```python
from build123d import *

# Parameters (mm, degrees)
EXTRUDE_1_DEPTH              = 88
HOLE_WIZARD_M4_1_D           = 4.5
HOLE_WIZARD_M4_1_CBORE_D     = 8
HOLE_WIZARD_M4_1_CBORE_DEPTH = 4.4
HOLE_WIZARD_M4_1_2_D         = 3.3
HOLE_WIZARD_M3_1_D           = 2.5
HOLE_WIZARD_M3_1_DEPTH       = 9.5
HOLE_WIZARD_M3_1_TIP         = 0.751075774
SKETCH_8_R                   = 1.75
CUT_EXTRUDE_1_DEPTH          = 5


with BuildPart() as part:
    # 草图1 → 凸台-拉伸1 (new body)
    with BuildSketch(Plane.XY):
        Polygon((-9, 10), (-9, 5), (-74, 5), (-74, 12), (-79, 12), (-79, 5.9), (-79.6, 5.9), (-79.6, 0), (0, 0), (0, 10), (-2, 10), (-2, 8), (-7, 8), (-7, 10), align=None)
    extrude(amount=EXTRUDE_1_DEPTH)

    # Hole Wizard M4 _1 (through all)
    with Locations(Plane(origin=(0, 0, 0), x_dir=(-1, 0, 0), z_dir=(0, -1, 0))):
        with Locations((4.5, -11.5), (4.5, -44), (4.5, -76.5)):
            CounterBoreHole(HOLE_WIZARD_M4_1_D / 2, HOLE_WIZARD_M4_1_CBORE_D / 2, HOLE_WIZARD_M4_1_CBORE_DEPTH)

    # Hole Wizard M4 _1 2 (through all)
    with Locations(Plane(origin=(0, 0, 0), x_dir=(-1, 0, 0), z_dir=(0, -1, 0))):
        with Locations((68.8, -14), (68.8, -22)):
            Hole(HOLE_WIZARD_M4_1_2_D / 2)

    # M3 螺纹孔1
    with Locations(Plane.ZY.offset(79.6)):
        with Locations((11.5, 3), (44, 3), (76.5, 3)):
            Hole(HOLE_WIZARD_M3_1_D / 2, depth=HOLE_WIZARD_M3_1_DEPTH)
            with Locations((0, 0, -(HOLE_WIZARD_M3_1_DEPTH + HOLE_WIZARD_M3_1_TIP / 2))):  # 118° drill point
                Cone(0, HOLE_WIZARD_M3_1_D / 2, HOLE_WIZARD_M3_1_TIP, mode=Mode.SUBTRACT)

    # 草图8 → 切除-拉伸1 (cut)
    with BuildSketch(Plane.ZY.offset(79)):
        with Locations((63, 9.5)):
            Circle(SKETCH_8_R)
    extrude(amount=-CUT_EXTRUDE_1_DEPTH, mode=Mode.SUBTRACT)


solid = part.part
```
Work out the finished part from the listing and answer in its coordinate system (mm). A direction names the side the tool comes from. Coordinates: 2 decimals unless noted, no trailing zeros. Write each loop counter-clockwise with the first axis right and the second up, starting at its lowest first coordinate (ties: lowest second). Pieces come first, ordered by that corner, then holes. Notation, with made-up numbers: (42.25, -38) - (70.25, -38) arc R14 cw to (70.25, -28) - close; hole circle Ø2 at (9, -13.5). An arc over 180 degrees is marked (long way). Answer as a JSON object with one key per item and string values.
Q1. Find section B-B (z = 34). Write down the section's boundary in (x, y), plus the area to 3 significant figures.
Results list:
{"outline": "(-79.6, 0) - (0, 0) - (0, 10) - (-2, 10) - (-2, 8) - (-7, 8) - (-7, 10) - (-9, 10) - (-9, 5) - (-74, 5) - (-74, 12) - (-79, 12) - (-79, 5.9) - (-79.6, 5.9) - close", "area": "469 mm^2"}
Q2. Consider L1, parallel to Z at x = -4.5, y = 6.2; L2, parallel to Z at x = -68.8, y = 2.05; L3, parallel to X at y = 8.25, z = 74. Determine where each line is inside the solid, lowest interval first. Write a range as from..to.
Results list:
{"L1": "z = 0..9.25, 13.75..41.75, 46.25..74.25, 78.75..88", "L2": "z = 0..12.35, 15.65..20.35, 23.65..88", "L3": "x = -79..-74, -9..-7, -2..0"}
Q3. For a pull along Z with two mould halves and no side action, classify faces 1 (the conical face through (-69.479, 2.868, 76.328)), 2 (the flat face through (0, 5, 43)), 3 (the flat face through (-40, 3, 0)) as pulls with the +Z half, pulls with the -Z half, needs draft (parallel to the pull), parting line crosses it, or undercut.
Results list:
{"face 1": "undercut", "face 2": "needs draft", "face 3": "pulls with the -Z half"}
Q4. Find section A-A (z = 63). Write down the section's boundary in (x, y).
Results list:
{"outline": "(-79.6, 0) - (0, 0) - (0, 10) - (-2, 10) - (-2, 8) - (-7, 8) - (-7, 10) - (-9, 10) - (-9, 5) - (-74, 5) - (-74, 7.75) - (-79, 7.75) - (-79, 5.9) - (-79.6, 5.9) - close; (-79, 11.25) - (-74, 11.25) - (-74, 12) - (-79, 12) - close"}
Q5. Find section C-C (x = -40). Write down the section's boundary in (y, z), plus the area to 3 significant figures.
Results list:
{"outline": "(0, 0) - (5, 0) - (5, 88) - (0, 88) - close", "area": "440 mm^2"}
Q6. Given pin 1 Ø1 at (x, z) = (-8.5, 29) entering from +Y; pin 2 Ø2.5 at (x, z) = (-6.5, 77) entering from -Y; pin 3 Ø1.5 at (x, z) = (-68, 46) entering from +Y, each flat-ended and moving along its own axis, determine where each tip first touches the part or whether it passes through.
Results list:
{"pin 1": "stops at y = 10", "pin 2": "stops at y = 4.4", "pin 3": "stops at y = 5"}
Q7. Which of the six approach directions +Z, -Z, +X, -X, +Y, -Y give full straight-line access (tool end or side, diameter ignored) to faces 4 (the cylindrical face through (-3.979, 2.169, 40.034)), 5 (the flat face through (-8, 10, 43)), 6 (the flat face through (-2, 9, 43))?
Results list:
{"face 4": "-Y", "face 5": "+Z, -Z, +X, +Y", "face 6": "+Z, -Z, +Y"}
